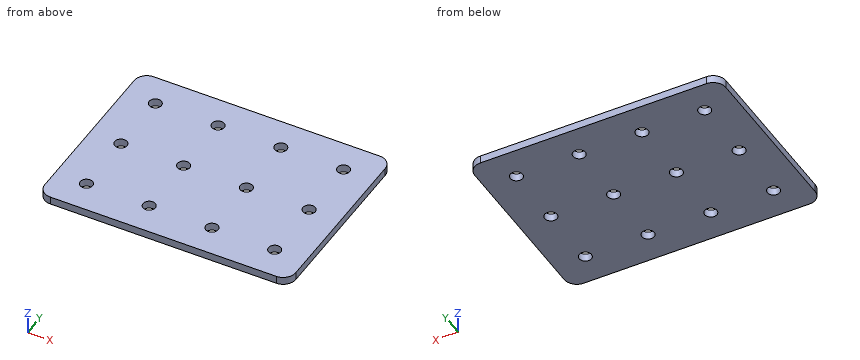
```python
from build123d import *

# Parameters (mm, degrees)
BOSS_EXTRUDE1_START = -3248.025
SKETCH1_R           = 2.5
BOSS_EXTRUDE1_DEPTH = 3.175


with BuildPart() as part:
    # Sketch1 → Boss-Extrude1 (new body)
    with BuildSketch(Plane.XY.offset(BOSS_EXTRUDE1_START)):
        with BuildLine():
            Line((71.12, 76.200000002), (-20.32, 76.200000002))
            ThreePointArc((-20.32, 76.200000002), (-23.912102448, 74.71210245), (-25.4, 71.120000002))
            Line((-25.4, 71.120000002), (-25.4, 5.08))
            ThreePointArc((-25.4, 5.08), (-23.912102448, 1.487897552), (-20.32, 0))
            Line((-20.32, 0), (71.12, 0))
            ThreePointArc((71.12, 0), (74.712102448, 1.487897552), (76.2, 5.08))
            Line((76.2, 5.08), (76.2, 71.120000002))
            ThreePointArc((76.2, 71.120000002), (74.712102448, 74.71210245), (71.12, 76.200000002))
        make_face()
        with Locations(Location((63.5, 63.5, 0), (0, 0, 90))):
            Circle(SKETCH1_R, mode=Mode.SUBTRACT)
        with Locations(Location((63.5, 38.1, 0), (0, 0, 90))):
            Circle(SKETCH1_R, mode=Mode.SUBTRACT)
        with Locations(Location((-12.7, 63.5, 0), (0, 0, 90))):
            Circle(SKETCH1_R, mode=Mode.SUBTRACT)
        with Locations(Location((12.7, 63.5, 0), (0, 0, 90))):
            Circle(SKETCH1_R, mode=Mode.SUBTRACT)
        with Locations(Location((38.1, 63.5, 0), (0, 0, 90))):
            Circle(SKETCH1_R, mode=Mode.SUBTRACT)
        with Locations(Location((-12.7, 38.1, 0), (0, 0, 90))):
            Circle(SKETCH1_R, mode=Mode.SUBTRACT)
        with Locations(Location((12.7, 38.1, 0), (0, 0, 90))):
            Circle(SKETCH1_R, mode=Mode.SUBTRACT)
        with Locations(Location((38.1, 38.1, 0), (0, 0, 90))):
            Circle(SKETCH1_R, mode=Mode.SUBTRACT)
        with Locations(Location((38.1, 12.7, 0), (0, 0, 90))):
            Circle(SKETCH1_R, mode=Mode.SUBTRACT)
        with Locations(Location((12.7, 12.7, 0), (0, 0, 90))):
            Circle(SKETCH1_R, mode=Mode.SUBTRACT)
        with Locations(Location((-12.7, 12.7, 0), (0, 0, 90))):
            Circle(SKETCH1_R, mode=Mode.SUBTRACT)
        with Locations(Location((63.5, 12.7, 0), (0, 0, 90))):
            Circle(SKETCH1_R, mode=Mode.SUBTRACT)
    extrude(amount=-BOSS_EXTRUDE1_DEPTH)


solid = part.part
```
Geometry check sheet. Reference: the model listing, model coordinates, mm. Coordinates: 2 decimals unless noted, no trailing zeros. Order: outer loops, then holes, each group sorted by start corner. A loop starts at its lowest first (then second) coordinate and runs counter-clockwise, first axis right, second up.
Q1. Sectioned sample at B-B on y = 63.5. Record the cut outline in (x, z) (3 decimals), and give its area (3 significant figures).
Reply:
outline: (-25.4, -3251.2) - (-15.2, -3251.2) - (-15.2, -3248.025) - (-25.4, -3248.025) - close; (-10.2, -3251.2) - (10.2, -3251.2) - (10.2, -3248.025) - (-10.2, -3248.025) - close; (15.2, -3251.2) - (35.6, -3251.2) - (35.6, -3248.025) - (15.2, -3248.025) - close; (40.6, -3251.2) - (61, -3251.2) - (61, -3248.025) - (40.6, -3248.025) - close; (66, -3251.2) - (76.2, -3251.2) - (76.2, -3248.025) - (66, -3248.025) - close
area: 259 mm2
Q2. Sectioned sample at C-C on z = -3250.2. Give the number of separate pieces and of enclosed holes in the cut face, and give its area (3 significant figures).
Reply:
separate pieces: 1
enclosed holes: 12
area: 7,480 mm2
Q3. Sectioned sample at A-A on x = -12.7. Record the cut outline in (y, z) (3 decimals), and give its area (3 significant figures).
Reply:
outline: (0, -3251.2) - (10.2, -3251.2) - (10.2, -3248.025) - (0, -3248.025) - close; (15.2, -3251.2) - (35.6, -3251.2) - (35.6, -3248.025) - (15.2, -3248.025) - close; (40.6, -3251.2) - (61, -3251.2) - (61, -3248.025) - (40.6, -3248.025) - close; (66, -3251.2) - (76.2, -3251.2) - (76.2, -3248.025) - (66, -3248.025) - close
area: 194 mm2
Q4. Thickness scan on probe 1 along X at (y, z) = (38.1, -3249.05); probe 2 along Y at (x, z) = (-13, -3250.55); probe 3 along Y at (x, z) = (11, -3250.65). Record the ranges inside material, lowest first.
Reply:
probe 1: x = -25.4 to -15.2, -10.2 to 10.2, 15.2 to 35.6, 40.6 to 61, 66 to 76.2
probe 2: y = 0 to 10.22, 15.18 to 35.62, 40.58 to 61.02, 65.98 to 76.2
probe 3: y = 0 to 10.87, 14.53 to 36.27, 39.93 to 61.67, 65.33 to 76.2
